from build123d import *

# Parameters (mm, degrees)
SKETCH_1_R             = 18.5
SKETCH_1_R_2           = 13
EXTRUDE_1_DEPTH        = 1.5
SKETCH_2_R             = 2.5
EXTRUDE_2_DEPTH        = 10.5
HOLE_WIZARD_M2_1_D     = 1.6
HOLE_WIZARD_M2_1_DEPTH = 7
HOLE_WIZARD_M2_1_TIP   = 0.480688495
SKETCH_4_OUTSIDE_W     = 49.736
SKETCH_4_OUTSIDE_H     = 49.736
CUT_EXTRUDE_1_DEPTH    = 10
FILLET_1_R             = 2


with BuildPart() as part:
    # 草图1 → 凸台-拉伸1 (new body)
    with BuildSketch(Plane(origin=(0, 0, 0), x_dir=(1, 0, 0), z_dir=(0, 1, 0))):
        with Locations(Location((0, 0, 0), (0, 0, 270))):
            Circle(SKETCH_1_R)
        with Locations(Location((0, 0, 0), (0, 0, 270))):
            Circle(SKETCH_1_R_2, mode=Mode.SUBTRACT)
    extrude(amount=EXTRUDE_1_DEPTH)

    # 草图2 → 凸台-拉伸2 (add)
    with BuildSketch(Plane(origin=(0, 1.5, 0), x_dir=(1, 0, 0), z_dir=(0, 1, 0))):
        with Locations(Location((15.75, 0, 0), (0, 0, 90))):
            Circle(SKETCH_2_R)
        with Locations(Location((-7.875, -13.63990011, 0), (0, 0, 90))):
            Circle(SKETCH_2_R)
        with Locations(Location((-7.875, 13.63990011, 0), (0, 0, 90))):
            Circle(SKETCH_2_R)
    extrude(amount=EXTRUDE_2_DEPTH)

    # M2 螺纹孔1
    with Locations(Plane(origin=(15.75, 12, 0), x_dir=(0, 0, 1), z_dir=(0, 1, 0))):
        with Locations((0, 0), (-13.63990011, -23.625), (13.63990011, -23.625)):
            Hole(HOLE_WIZARD_M2_1_D / 2, depth=HOLE_WIZARD_M2_1_DEPTH)
            with Locations((0, 0, -(HOLE_WIZARD_M2_1_DEPTH + HOLE_WIZARD_M2_1_TIP / 2))):  # 118° drill point
                Cone(0, HOLE_WIZARD_M2_1_D / 2, HOLE_WIZARD_M2_1_TIP, mode=Mode.SUBTRACT)

    # 草图4 outside → 切除-拉伸1 (cut)
    with BuildSketch(Plane(origin=(0, 1.5, 0), x_dir=(1, 0, 0), z_dir=(0, 1, 0))):
        Rectangle(SKETCH_4_OUTSIDE_W, SKETCH_4_OUTSIDE_H)
        with BuildLine():
            ThreePointArc((16.583333333, 2.357022604), (8.375, 14.505925513), (-6.250425214, 15.540099248))
            ThreePointArc((-6.250425214, 15.540099248), (-9.125, 15.804963619), (-10.332908119, 13.183076644))
            ThreePointArc((-10.332908119, 13.183076644), (-16.75, 0), (-10.332908119, -13.183076644))
            ThreePointArc((-10.332908119, -13.183076644), (-9.125, -15.804963619), (-6.250425214, -15.540099248))
            ThreePointArc((-6.250425214, -15.540099248), (8.375, -14.505925513), (16.583333333, -2.357022604))
            ThreePointArc((16.583333333, -2.357022604), (18.25, 0), (16.583333333, 2.357022604))
        make_face(mode=Mode.SUBTRACT)
    extrude(amount=-CUT_EXTRUDE_1_DEPTH, mode=Mode.SUBTRACT)

    # 圆角1
    fillet_1_edges = [part.edges().sort_by_distance(p)[0] for p in [
        (-6.250425214, 0.75, 15.540099248),
        (-10.332908119, 0.75, 13.183076644),
        (-10.332908119, 0.75, -13.183076644),
        (-6.250425214, 0.75, -15.540099248),
        (16.583333333, 0.75, -2.357022604),
        (16.583333333, 0.75, 2.357022604),
    ]]
    fillet(fillet_1_edges, radius=FILLET_1_R)


solid = part.part
The listing builds one solid part. Answer for the finished solid, in the listing's coordinates (mm). A direction names the side the tool comes from. Coordinates: 2 decimals unless noted, no trailing zeros. Loops run counter-clockwise (first coordinate to the right, second up) from the corner with the lowest first, then second, coordinate; pieces in that order, holes last.
1) Find section B-B on z = 10.5. Write down the section's boundary in (x, y).
2) Determine the mould class of faces 1 (the face through (-16.75, 0.76, -0.2)), 2 (the face through (-12.3, 1.5, 4.9)), 3 (the face through (-7.76, 4.6, 13.71)) for opening direction X: pulls with the +X half, pulls with the -X half, needs draft (parallel to the pull), parting line crosses it, or undercut.
3) Find section C-C on x = -13.5. Write down the section's boundary in (y, z), then the cut area to 3 significant figures.
4) Flat-ended cylindrical pins translate along their axes: pin 1 Ø4 at (x, y) = (-3, 4.5) entering from +Z; pin 2 Ø1.3 at (x, z) = (-7.88, 13.64) entering from +Y; pin 3 Ø1 at (y, z) = (10.5, -1) entering from -X. Find the tip coordinate at first contact, or state that the pin passes through.
5) Find the intervals of material crossed by L1, parallel to X at y = 1.15, z = 0; L2, parallel to Z at x = 15.75, y = 6.5; L3, parallel to Y at x = -14.5, z = -5, in increasing order.
6) A tool of negligible diameter and unlimited length cuts with its end or side. For faces 4 (the face through (14.97, 8.45, 0.17)), 5 (the face through (8.201, 0.76, 14.605)), from which of +Z, -Z, +X, -X, +Y, -Y can it reach the whole face along a straight path? Write none if from no direction.
7) Find section A-A on x = 0. Write down the section's boundary in (y, z).
Values:
1. outline: (-13.05, 0) - (-7.66, 0) - (-7.66, 1.5) - (-13.05, 1.5) - close; (7.66, 0) - (13.05, 0) - (13.05, 1.5) - (7.66, 1.5) - close
2. face 1: pulls with the -X half
2. face 2: needs draft
2. face 3: undercut
3. outline: (0, -9.92) - (1.5, -9.92) - (1.5, 9.92) - (0, 9.92) - close
3. area: 29.7 mm2
4. pin 1: passes through
4. pin 2: stops at y = 4.91
4. pin 3: stops at x = 13.3
5. L1: x = -16.75 to -13, 13 to 18.25
5. L2: z = -2.5 to -0.8, 0.8 to 2.5
5. L3: y = 0 to 1.5
6. face 4: +Y
6. face 5: +Z, +Y, -Y
7. outline: (0, -16.75) - (1.5, -16.75) - (1.5, -13) - (0, -13) - close; (0, 13) - (1.5, 13) - (1.5, 16.75) - (0, 16.75) - close
